Geometry: final body of the model. Coordinates: model frame, mm. A direction names the side the tool comes from. Round coordinates to 2 decimals unless told otherwise and drop trailing zeros. Loops run counter-clockwise (first coordinate to the right, second up) from the corner with the lowest first, then second, coordinate; pieces in that order, holes last. Notation, with made-up numbers: (-15.5, 64) - (-11.5, 64) arc R32 ccw to (-11.5, 101) - close; hole circle Ø5 at (19, 52.5). An arc over 180 degrees is marked (long way). Return JSON: item names as keys, results as strings. Group by question number.
1. Section A-A on z = 5. Return loops of the section in (x, y), and give its area (3 significant figures).
2. Material intervals for probe 1 along X at (y, z) = (6.75, 5); probe 2 along Y at (x, z) = (-20.5, 0.5); probe 3 along Y at (x, z) = (3, 7.25), sorted ascending.
3. Set-up query: faces 1 (the face through (-1, 10, 3)), 2 (the face through (13.138, 1.848, 0.21)), 3 (the face through (0, 24, -5)). Return all of +Z, -Z, +X, -X, +Y, -Y with unobstructed straight access to the full face (end or side cutting, diameter ignored); none if empty.
4. Section C-C on y = 5.5. Return loops of the section in (x, z).
5. Draft query along X for faces 4 (the face through (14.248, 21.373, -14.287)), 5 (the face through (-4, 26, -9.7)), 6 (the face through (-4.155, 22.011, -12.387)), 7 (the face through (-15, 21, -10)). Return one class per face: +X half, -X half, draft (parallel to the pull), parting line (faces both ways), or undercut.
6. Section B-B on x = -30. Return loops of the section in (y, z), and give its area (3 significant figures).
7. First-contact query: pin 1 Ø4 at (y, z) = (10.5, -7.5) entering from +X; pin 2 Ø20 at (x, y) = (-2, 34.5) entering from +Z; pin 3 Ø1.5 at (y, z) = (23.5, -10.5) entering from -X. Flat tips, straight axial feed; report the tip coordinate or a pass-through.
8. Section D-D on y = 20. Return loops of the section in (x, z).
from build123d import *

# Parameters (mm, degrees)
SKETCH1_W                               = 80
SKETCH1_H                               = 30
BOSS_EXTRUDE1_DEPTH                     = 10
BOSS_EXTRUDE2_DEPTH                     = 10
SKETCH4_R                               = 15
BOSS_EXTRUDE3_DEPTH                     = 10
CBORE_FOR_M5_HEX_HEAD_BOLT1_D           = 9
CBORE_FOR_M5_HEX_HEAD_BOLT1_CBORE_D     = 18.01
CBORE_FOR_M5_HEX_HEAD_BOLT1_CBORE_DEPTH = 5.3
CUT_EXTRUDE1_REACH                      = 69.268
SKETCH7_W                               = 30
SKETCH7_H                               = 2.5
CUT_EXTRUDE2_REACH                      = 57.227
SKETCH8_R                               = 5
FILLET1_R                               = 5
FILLET2_R                               = 2.5


with BuildPart() as part:
    # Sketch1 → Boss-Extrude1 (new body)
    with BuildSketch(Plane(origin=(0, 0, 0), x_dir=(1, 0, 0), z_dir=(0, 1, 0))):
        Rectangle(SKETCH1_W, SKETCH1_H)
    extrude(amount=BOSS_EXTRUDE1_DEPTH)

    # Sketch2 → Boss-Extrude2 (add)
    with BuildSketch(Plane(origin=(0, 0, -15), x_dir=(-1, 0, 0), z_dir=(0, 0, -1))):
        Polygon((0, 30), (15, 30), (15, 0), (-15, 0), (-15, 30), align=None)
    extrude(amount=-BOSS_EXTRUDE2_DEPTH)

    # Sketch4 → Boss-Extrude3 (add)
    with BuildSketch(Plane(origin=(0, 0, -15), x_dir=(-1, 0, 0), z_dir=(0, 0, -1))):
        with Locations((0, 30)):
            Circle(SKETCH4_R)
    extrude(amount=-BOSS_EXTRUDE3_DEPTH)

    # CBORE for M5 Hex Head Bolt1 (through all)
    with Locations(Plane(origin=(0, 0, -15), x_dir=(-1, 0, 0), z_dir=(0, 0, -1))):
        with Locations((0, 30)):
            CounterBoreHole(CBORE_FOR_M5_HEX_HEAD_BOLT1_D / 2, CBORE_FOR_M5_HEX_HEAD_BOLT1_CBORE_D / 2, CBORE_FOR_M5_HEX_HEAD_BOLT1_CBORE_DEPTH)

    # Sketch7 → Cut-Extrude1 (cut, up to next)
    with BuildSketch(Plane.XY.offset(15), mode=Mode.PRIVATE) as cut_extrude1_sk1:
        with Locations((0, 1.25)):
            Rectangle(SKETCH7_W, SKETCH7_H)
    cut_extrude1_tool1 = extrude(cut_extrude1_sk1.sketch, amount=-CUT_EXTRUDE1_REACH, mode=Mode.PRIVATE) & part.part
    add(cut_extrude1_tool1.solids().sort_by_distance((0, 1.25, 15))[0], mode=Mode.SUBTRACT)

    # Sketch8 → Cut-Extrude2 (cut, up to next)
    with BuildSketch(Plane(origin=(0, 10, 0), x_dir=(1, 0, 0), z_dir=(0, 1, 0)), mode=Mode.PRIVATE) as cut_extrude2_sk1:
        with Locations(Location((-30, -5, 0), (0, 0, 270))):
            Circle(SKETCH8_R)
    cut_extrude2_tool1 = extrude(cut_extrude2_sk1.sketch, amount=-CUT_EXTRUDE2_REACH, mode=Mode.PRIVATE) & part.part
    # Sketch8 → Cut-Extrude2 (cut, up to next)
    with BuildSketch(Plane(origin=(0, 10, 0), x_dir=(1, 0, 0), z_dir=(0, 1, 0)), mode=Mode.PRIVATE) as cut_extrude2_sk2:
        with Locations(Location((30, -5, 0), (0, 0, 270))):
            Circle(SKETCH8_R)
    cut_extrude2_tool2 = extrude(cut_extrude2_sk2.sketch, amount=-CUT_EXTRUDE2_REACH, mode=Mode.PRIVATE) & part.part
    add(cut_extrude2_tool1.solids().sort_by_distance((-30, 10, 5))[0], mode=Mode.SUBTRACT)
    add(cut_extrude2_tool2.solids().sort_by_distance((30, 10, 5))[0], mode=Mode.SUBTRACT)

    # Fillet1
    # the kernel refuses this fillet: 5 mm, written as the material it adds along each edge
    with BuildSketch(Plane(origin=(15, 2.5, 15), x_dir=(-1, 0, 0), z_dir=(0, 0, -1))) as fillet1_piece_1:
        with BuildLine():
            CenterArc((4.330127019, -5), FILLET1_R, 90, 60)
            Line((0, -2.5), (0, 0))
            Line((0, 0), (4.330127019, 0))
        make_face()
    extrude(amount=30)
    with BuildSketch(Plane(origin=(-15, 2.5, 15), x_dir=(0, -1, 0), z_dir=(0, 0, -1))) as fillet1_piece_2:
        with BuildLine():
            CenterArc((5, -4.330127019), FILLET1_R, 120, 60)
            Line((0, -4.330127019), (0, 0))
            Line((0, 0), (2.5, 0))
        make_face()
    extrude(amount=30)
    # the kernel refuses this fillet: 5 mm, written as the material it takes off along each edge
    with BuildSketch(Plane(origin=(-40, -12.5, -15), x_dir=(0, 0, 1), z_dir=(0, 1, 0)), Plane(origin=(-40, -12.5, 15), x_dir=(1, 0, 0), z_dir=(0, 1, 0))) as fillet1_2_piece_1:
        with BuildLine():
            CenterArc((FILLET1_R, FILLET1_R), FILLET1_R, 180, 90)
            Line((0, FILLET1_R), (0, 0))
            Line((0, 0), (FILLET1_R, 0))
        make_face()
    extrude(amount=35, mode=Mode.SUBTRACT)
    with BuildSketch(Plane(origin=(40, -12.5, -15), x_dir=(0, 0, 1), z_dir=(0, 1, 0)), Plane(origin=(40, -12.5, 15), x_dir=(-1, 0, 0), z_dir=(0, 1, 0))) as fillet1_2_piece_2:
        with BuildLine():
            CenterArc((FILLET1_R, -FILLET1_R), FILLET1_R, 90, 90)
            Line((0, -FILLET1_R), (0, 0))
            Line((0, 0), (FILLET1_R, 0))
        make_face()
    extrude(amount=35, mode=Mode.SUBTRACT)

    # Fillet2
    fillet2_edges = [part.edges().sort_by_distance(p)[0] for p in [
        (-25, 10, -15),
        (-15, 20, -5),
        (15, 10, -10),
        (15, 20, -15),
        (15, 20, -5),
        (-15, 20, -15),
        (-15, 10, -10),
        (0, 10, -5),
        (0, 45, -15),
        (0, 45, -5),
        (-40, 10, 0),
        (25, 10, -15),
        (0, 10, 15),
        (40, 10, 0),
        (38.535533906, 10, 13.535533906),
        (38.535533906, 10, -13.535533906),
        (-38.535533906, 10, 13.535533906),
        (-38.535533906, 10, -13.535533906),
    ]]
    fillet(fillet2_edges, radius=FILLET2_R)


solid = part.part
Taken from the geometry:
{
 "1": {"outline": "(-40, 0) - (-35, 0) - (-35, 10) - (-37.5, 10) arc R2.5 ccw to (-40, 7.5) - close; (-25, 0) - (-15, 0) arc R5 cw to (-10.67, 2.5) - (10.67, 2.5) arc R5 cw to (15, 0) - (25, 0) - (25, 10) - (-25, 10) - close; (35, 0) - (40, 0) - (40, 7.5) arc R2.5 ccw to (37.5, 10) - (35, 10) - close", "area": "529 mm2"},
 "2": {"probe 1": "-40 to -35, -25 to 25, 35 to 40", "probe 2": "0 to 10", "probe 3": "2.5 to 10"},
 "3": {"face 1": "+Z, +Y", "face 2": "+Z, -Z, -Y", "face 3": "+Z, +X, -X, +Y"},
 "4": {"outline": "(-40, -10) arc R5 ccw to (-35, -15) - (35, -15) arc R5 ccw to (40, -10) - (40, 10) arc R5 ccw to (35, 15) - (-35, 15) arc R5 ccw to (-40, 10) - close; hole circle Ø10 at (-30, 5); hole circle Ø10 at (30, 5)"},
 "5": {"face 4": "+X half", "face 5": "undercut", "face 6": "undercut", "face 7": "-X half"},
 "6": {"outline": "(0, -15) - (7.5, -15) arc R2.5 ccw to (10, -12.5) - (10, 0) - (0, 0) - close; (0, 10) - (10, 10) - (10, 12.5) arc R2.5 ccw to (7.5, 15) - (0, 15) - close", "area": "197 mm2"},
 "7": {"pin 1": "x = 39.79", "pin 2": "z = -5", "pin 3": "x = -15"},
 "8": {"outline": "(-15, -12.5) arc R2.5 ccw to (-12.5, -15) - (12.5, -15) arc R2.5 ccw to (15, -12.5) - (15, -7.5) arc R2.5 ccw to (12.5, -5) - (-12.5, -5) arc R2.5 ccw to (-15, -7.5) - close"}
}
